```python
from build123d import *

# Parameters (mm, degrees)
F0_W      = 152.4
F0_H      = 88.9
F1_DEPTH  = 2.54
F3_DEPTH  = 12.7
F4_W      = 127
F4_H      = 1.27
F5_DEPTH  = 5.08
F6_W      = 146.05
F6_H      = 9.525
F7_DEPTH  = 22.86
F8_R      = 2.54
F9_DEPTH  = 2.541
F10_W     = 152.4
F10_H     = 2.54
F11_DEPTH = 9.525
F12_ANGLE = 30


with BuildPart() as f1:
    # F0 (on Top) → F1 (new body)
    with BuildSketch(Plane.XY):
        Rectangle(F0_W, F0_H)
    extrude(amount=F1_DEPTH)

    # F2 (on face) → F3 (join)
    with BuildSketch(Plane.XY.offset(2.54)):
        Polygon((63.5, -41.91), (-63.5, -41.91), (-63.5, -19.05), (-76.2, -19.05), (-76.2, -44.45), (76.2, -44.45), (76.2, -19.05), (63.5, -19.05), align=None)
    extrude(amount=F3_DEPTH)

    # F4 (on face) → F5 (join)
    with BuildSketch(Plane(origin=(0, -41.91, 0), x_dir=(-1, 0, 0), z_dir=(0, 1, 0))):
        with Locations((0, 14.605)):
            Rectangle(F4_W, F4_H)
    extrude(amount=F5_DEPTH)

    # F6 (on face) → F7 (cut, through all)
    with BuildSketch(Plane(origin=(0, -19.05, 0), x_dir=(-1, 0, 0), z_dir=(0, 1, 0))):
        with Locations((0, 7.3025)):
            Rectangle(F6_W, F6_H)
    extrude(amount=-F7_DEPTH, mode=Mode.SUBTRACT)

    # F8 (on face) → F9 (cut, through all)
    with BuildSketch(Plane.XY.offset(2.54)):
        with Locations((0, 38.1)):
            Circle(F8_R)
        with Locations((-63.5, 38.1)):
            Circle(F8_R)
        with Locations((63.5, 38.1)):
            Circle(F8_R)
    extrude(amount=-F9_DEPTH, mode=Mode.SUBTRACT)

    # F10 (on face) → F11 (join)
    with BuildSketch(Plane(origin=(0, 0, 0), x_dir=(1, 0, 0), z_dir=(0, 0, -1))):
        with Locations((0, 43.18)):
            Rectangle(F10_W, F10_H)
    extrude(amount=F11_DEPTH)


with BuildPart() as f1_1:
    # F12: moved
    add(f1.part.rotate(Axis((-76.2, 12.7, 2.54), (0, 1, 0)), F12_ANGLE))


solid = f1_1.part
```
The model under review builds one solid part; all positions refer to its coordinate system, in mm. A direction names the side the tool comes from. Round coordinates to 2 decimals unless told otherwise and drop trailing zeros. Loops run counter-clockwise (first coordinate to the right, second up) from the corner with the lowest first, then second, coordinate; pieces in that order, holes last. Notation, with made-up numbers: M -1,-13 L 8,-13 A27 cw 8,21 Z; hole C 30.5,-8.75 d6. An arc over 180 degrees is marked long. Write item = value, one per line.
Item 1: Machinability: for faces 1 (the flat face through (-12.4, 1.87, -37.23)), 2 (the cylindrical face through (-9.65, 40.24, -37.33)), 3 (the flat face through (58, -19.05, -63)), 4 (the flat face through (55.38, -30.32, -68.01)), 5 (the flat face through (-11, -44.45, -35)), which of the approach directions +Z, -Z, +X, -X, +Y, -Y give a long, thin tool a straight path to every point of the face, cutting with its end or side? Answer none if there is none.
Return value:
face_1 = -Z, -X, +Y
face_2 = none
face_3 = +Z, +X, +Y
face_4 = +Y
face_5 = +Z, -Z, +X, -X, -Y
Item 2: Take a section at A-A on z = -45.5. Write out the cut boundary in (x, y).
Return value:
outline = M -17.12,-44.45 L 32.41,-44.45 L 32.41,-36.83 L 29.87,-36.83 L 29.87,-41.91 L 7.01,-41.91 L 7.01,44.45 L 1.93,44.45 L 1.93,-41.91 L -17.12,-41.91 Z
Item 3: Take a section at B-B on y = 28.5. Write out the cut boundary in (x, z), then the cut area to 3 significant figures.
Return value:
outline = M -77.47,0.34 L 54.51,-75.86 L 55.78,-73.66 L -76.2,2.54 Z
area = 387 mm2
Item 4: The part is to be moulded in two halves that separate along X. For faces 6 (the flat face through (-17.165, -43.198, -45.475)), 7 (the flat face through (-15, -41.91, -41)), 8 (the cylindrical face through (-64.645, 40.242, -5.577)), 9 (the flat face through (-64.51, -30.32, 6.79)), say which applies: released by +X, released by -X, zero draft, split by the parting line, or undercut.
Return value:
face_6 = released by -X
face_7 = zero draft
face_8 = undercut
face_9 = undercut
Item 5: Take a section at C-C on x = 25. Write out the cut boundary in (y, z), then the cut area to 3 significant figures.
Return value:
outline = M -44.45,-69.82 L -41.91,-69.82 L -41.91,-58.82 L 44.45,-58.82 L 44.45,-55.89 L -41.91,-55.89 L -41.91,-42.69 L -36.83,-42.69 L -36.83,-41.22 L -44.45,-41.22 Z
area = 333 mm2
Item 6: Insertion check: P1, Ø10, axis at x = 57.5, z = -62, coming from the +Y side; P2, Ø8, axis at x = 43, y = -23, coming from the +Z side; P3, Ø12, axis at y = -23.5, z = -41, coming from the +X side. Each pin has a flat end and moves straight along its axis. Give the tip position at first contact, or say it passes through.
Return value:
P1 = -19.05
P2 = -63.97
P3 = 9.61
Item 7: For line 1 (X direction, y = -40, z = -46); line 2 (Y direction, x = 7, z = -49); line 3 (Z direction, x = 28, y = -41), list the stretches that pass through material, from the lowest coordinate up. Write a range as [from, to].
Return value:
line_1 = [2.79, 7.87], [30.73, 33.27]
line_2 = [-44.45, -41.91]
line_3 = [-60.55, -57.62], [-44.42, -42.96]
